Verification items for the finished model (mm, model axes). Give positions to 0.01 mm unless a question says otherwise; leave off trailing zeros. Loops run counter-clockwise (first coordinate to the right, second up) from the corner with the lowest first, then second, coordinate; pieces in that order, holes last. Notation, with made-up numbers: M 84.25,2 L 95.25,2 A20 cw 95.25,24 Z; hole C 53.5,-27.5 d1. An arc over 180 degrees is marked long. Answer in a Markdown table with one row per item.
```python
from build123d import *

# Parameters (mm, degrees)
SKETCH_1_W            = 426
SKETCH_1_H            = 40
EXTRUDE_1_DEPTH       = 3.7
SKETCH_1_2_W          = 426
SKETCH_1_2_H          = 40
SKETCH_1_2_W_2        = 422.8
SKETCH_1_2_H_2        = 36.8
CUT_EXTRUDE_1_DEPTH   = 1.2
SKETCH_2_R            = 2.75
SKETCH_2_R_2          = 1.15
SKETCH_2_R_3          = 3.006394209
SKETCH_2_W            = 27.5
SKETCH_2_H            = 19.5
CUT_EXTRUDE_1_2_DEPTH = 6
FILLET_1_R            = 2


with BuildPart() as part:
    # Sketch 1 → Extrude 1 (new body)
    with BuildSketch(Plane(origin=(0, 0, 0), x_dir=(1, 0, 0), z_dir=(0, 1, 0))):
        Rectangle(SKETCH_1_W, SKETCH_1_H)
    extrude(amount=EXTRUDE_1_DEPTH)

    # Sketch 1_2 → Cut-Extrude 1 (cut)
    with BuildSketch(Plane(origin=(0, 0, 0), x_dir=(1, 0, 0), z_dir=(0, 1, 0))):
        Rectangle(SKETCH_1_2_W, SKETCH_1_2_H)
        Rectangle(SKETCH_1_2_W_2, SKETCH_1_2_H_2, mode=Mode.SUBTRACT)
    extrude(amount=CUT_EXTRUDE_1_DEPTH, mode=Mode.SUBTRACT)

    # Sketch 2 → Cut-Extrude 1 2 (cut)
    with BuildSketch(Plane(origin=(0, 0, 0), x_dir=(1, 0, 0), z_dir=(0, 1, 0))):
        with Locations(Location((173, -9.5, 0), (0, 0, 270))):
            Circle(SKETCH_2_R)
        with Locations(Location((173, 9.5, 0), (0, 0, 270))):
            Circle(SKETCH_2_R)
        with Locations(Location((-179.25, 0, 0), (0, 0, 270))):
            Circle(SKETCH_2_R_2)
        with Locations(Location((-139.25, 0, 0), (0, 0, 270))):
            Circle(SKETCH_2_R_2)
        with Locations(Location((113, 9.5, 0), (0, 0, 270))):
            Circle(SKETCH_2_R_3)
        with Locations(Location((113, -9.5, 0), (0, 0, 270))):
            Circle(SKETCH_2_R_3)
        with Locations(Location((-9.9, -8.35, 0), (0, 0, 270))):
            Circle(SKETCH_2_R_2)
        with Locations(Location((-36.1, 8.35, 0), (0, 0, 270))):
            Circle(SKETCH_2_R_2)
        with Locations((-159.25, 0)):
            Rectangle(SKETCH_2_W, SKETCH_2_H)
        with BuildLine():
            ThreePointArc((-10.861951827, -2.986266323), (-12.07669601, 6.077123492), (-19.13728757, 11.888206454))
            ThreePointArc((-19.13728757, 11.888206454), (-21.657434592, 10.60412741), (-20.373355548, 8.083980389))
            ThreePointArc((-20.373355548, 8.083980389), (-15.572153287, 4.132443975), (-14.746127242, -2.0306611))
            ThreePointArc((-14.746127242, -2.0306611), (-13.281842146, -4.450551419), (-10.861951827, -2.986266323))
        make_face()
        with BuildLine():
            ThreePointArc((-26.86271243, 11.888206454), (-33.92330399, 6.077123492), (-35.138048173, -2.986266323))
            ThreePointArc((-35.138048173, -2.986266323), (-32.718157854, -4.450551419), (-31.253872758, -2.0306611))
            ThreePointArc((-31.253872758, -2.0306611), (-30.427846713, 4.132443975), (-25.626644452, 8.083980389))
            ThreePointArc((-25.626644452, 8.083980389), (-24.342565408, 10.60412741), (-26.86271243, 11.888206454))
        make_face()
        with BuildLine():
            ThreePointArc((-31.609426427, -9.062437674), (-23.135416387, -12.499266475), (-14.588935276, -9.246836768))
            ThreePointArc((-14.588935276, -9.246836768), (-14.455211749, -6.421572529), (-17.280475988, -6.287849002))
            ThreePointArc((-17.280475988, -6.287849002), (-23.092083143, -8.499501203), (-28.854409971, -6.162457618))
            ThreePointArc((-28.854409971, -6.162457618), (-31.681908227, -6.234939418), (-31.609426427, -9.062437674))
        make_face()
    extrude(amount=CUT_EXTRUDE_1_2_DEPTH, mode=Mode.SUBTRACT)

    # Fillet 1
    fillet_1_edges = [part.edges().sort_by_distance(p)[0] for p in [
        (-173, 1.85, -9.75),
        (-173, 1.85, 9.75),
        (-145.5, 1.85, 9.75),
        (-145.5, 1.85, -9.75),
    ]]
    fillet(fillet_1_edges, radius=FILLET_1_R)


solid = part.part
```
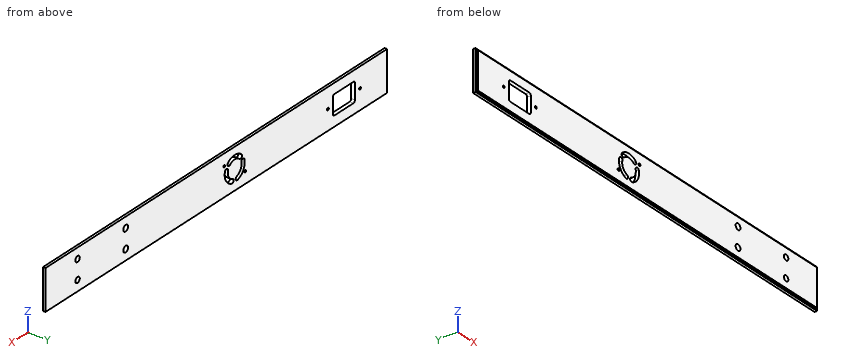
Item 1: Sectioned sample at A-A (x = -155.5). Record the cut outline in (y, z), and give its area (3 significant figures).
Reported:
| item | result |
|---|---|
| outline | M 0,-18.4 L 1.2,-18.4 L 1.2,-20 L 3.7,-20 L 3.7,-9.75 L 0,-9.75 Z; M 0,9.75 L 3.7,9.75 L 3.7,20 L 1.2,20 L 1.2,18.4 L 0,18.4 Z |
| area | 72.0 mm^2 |
Item 2: Sectioned sample at B-B (y = 2.55). State how many separate pieces and enclosed holes the cut face has, and give its area (3 significant figures).
Reported:
| item | result |
|---|---|
| separate pieces | 1 |
| enclosed holes | 12 |
| area | 16,200 mm^2 |
Item 3: Scan lines: L1, parallel to Z at x = 113, y = 0.95; L2, parallel to Z at x = 113, y = 2.8; L3, parallel to X at y = 1.9, z = 5. Record each from-to range of solid material in increasing order. Write a range as [from, to].
Reported:
| item | result |
|---|---|
| L1 | z = [-18.4, -12.51], [-6.49, 6.49], [12.51, 18.4] |
| L2 | z = [-20, -12.51], [-6.49, 6.49], [12.51, 20] |
| L3 | x = [-213, -173], [-145.5, 213] |
Item 4: Sectioned sample at C-C (x = -1). Record the cut outline in (y, z).
Reported:
| item | result |
|---|---|
| outline | M 0,-18.4 L 1.2,-18.4 L 1.2,-20 L 3.7,-20 L 3.7,20 L 1.2,20 L 1.2,18.4 L 0,18.4 Z |
Item 5: Go/stop test with flat-tipped pins: pin 1 (5.5 mm diameter, centred on x = 113, z = 9.5, fed in from -Y); pin 2 (7 mm diameter, centred on x = 113, z = -9.5, fed in from -Y); pin 3 (1.3 mm diameter, centred on y = 0.5, z = 3.5, fed in from -X); pin 4 (0.6 mm diameter, centred on y = 0.5, z = 5, fed in from +X). Record where each tip stops, or that it passes through.
Reported:
| item | result |
|---|---|
| pin 1 | passes through |
| pin 2 | stops at y = 0 |
| pin 3 | stops at x = -211.4 |
| pin 4 | stops at x = 211.4 |
